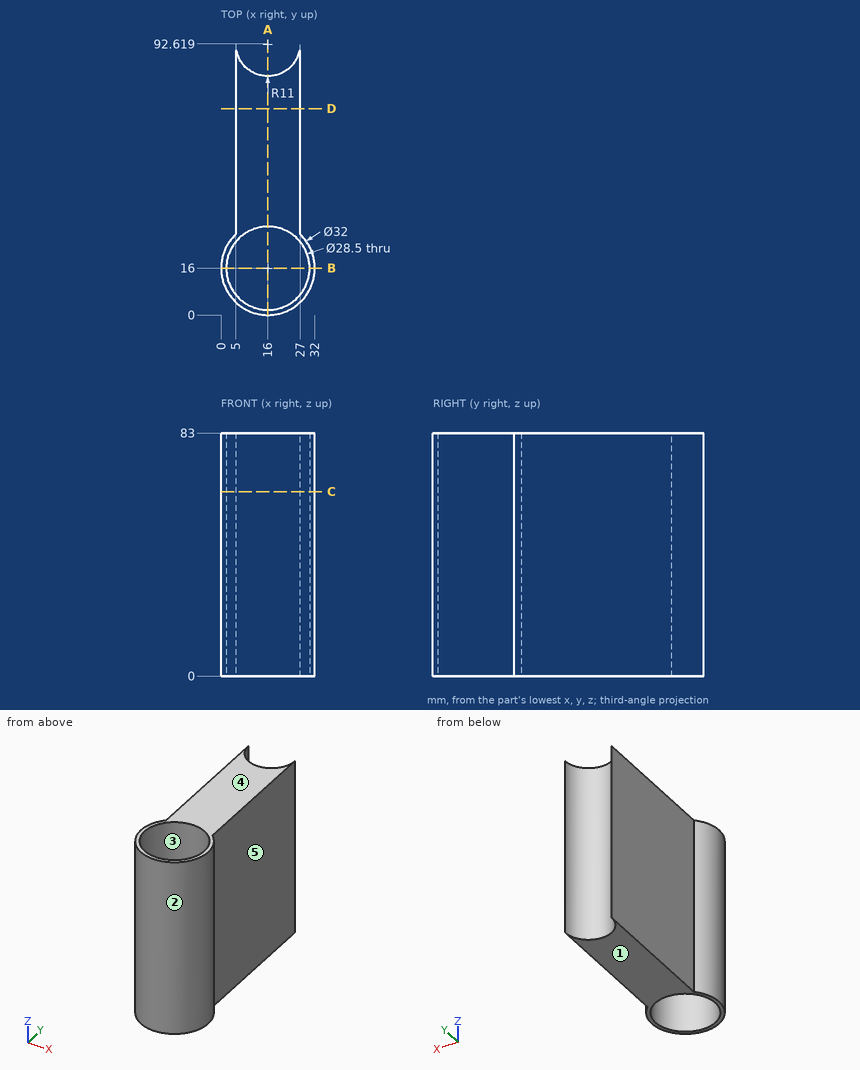
Design review of the part shown in the three views and the two pictorial views. Dimensions are in mm from the part's minimum x, y and z. A direction names the side the tool comes from. Coordinates: 2 decimals unless noted, no trailing zeros. Loops run counter-clockwise (first coordinate to the right, second up) from the corner with the lowest first, then second, coordinate; pieces in that order, holes last. Notation, with made-up numbers: (27.25, 75) -> (82.25, 75) arc R25 cw to (82.25, 87) -> close; hole circle Ø3 at (44.25, -36.5). An arc over 180 degrees is marked (long way). Answer as CSV lines item,"result".
Item 1: Take a section at D-D, the plane y = 70.5. State the section outline as (x, z) points, and give its area (3 significant figures).
Results below:
outline,"(5, 0) -> (27, 0) -> (27, 83) -> (5, 83) -> close"
area,"1,830 mm2"
Item 2: For L1, parallel to X at y = 16, z = 57.5; L2, parallel to Y at x = 16, z = 53; L3, parallel to X at y = 12.5, z = 47.5, list the stretches that pass through material, from the lowest coordinate up.
Results below:
L1,"x = 0 to 1.75, 30.25 to 32"
L2,"y = 0 to 1.75, 30.25 to 81.62"
L3,"x = 0.39 to 2.19, 29.81 to 31.61"
Item 3: Draft analysis for pull direction Y (two halves, no side actions). For the marked faces 1, 2 and 3, state which applies: +Y half, -Y half, draft (parallel to the pull), parting line (faces both ways), or undercut.
Results below:
face 1,"draft"
face 2,"parting line"
face 3,"undercut"
Item 4: Take a section at C-C, the plane z = 63. State the section outline as (x, y) points.
Results below:
outline,"(5, 27.62) arc R16 ccw (long way) to (27, 27.62) -> (27, 92.62) arc R11 cw to (5, 92.62) -> close; hole circle Ø28.5 at (16, 16)"
Item 5: Machinability: for the marked faces 4 and 5, which of the approach directions +Z, -Z, +X, -X, +Y, -Y give a long, thin tool a straight path to every point of the face, cutting with its end or side? Answer none if there is none.
Results below:
face 4,"+Z, +X, -X, +Y, -Y"
face 5,"+Z, -Z, +X, +Y"
Item 6: Insertion check: pin 1 (10 mm diameter, centred on y = 66, z = 29.5, fed in from +X); pin 2 (2 mm diameter, centred on x = 10, z = 20.5, fed in from +Y); pin 3 (12 mm diameter, centred on y = 42, z = 55, fed in from -X). Each pin has a flat end and moves straight along its axis. Give the tip position at first contact, or say it passes through.
Results below:
pin 1,"stops at x = 27"
pin 2,"stops at y = 84.13"
pin 3,"stops at x = 5"
Item 7: Take a section at A-A, the plane x = 16. State the section outline as (y, z) points.
Results below:
outline,"(0, 0) -> (1.75, 0) -> (1.75, 83) -> (0, 83) -> close; (30.25, 0) -> (81.62, 0) -> (81.62, 83) -> (30.25, 83) -> close"
Item 8: Take a section at B-B, the plane y = 16. State the section outline as (x, z) points.
Results below:
outline,"(0, 0) -> (1.75, 0) -> (1.75, 83) -> (0, 83) -> close; (30.25, 0) -> (32, 0) -> (32, 83) -> (30.25, 83) -> close"
